Read the model definition and answer for the solid it produces. Units are mm, in the model's axes. Face numbers are marked on the shaded views. A direction names the side the tool comes from. Round coordinates to 2 decimals unless told otherwise and drop trailing zeros. Write each loop counter-clockwise with the first axis right and the second up, starting at its lowest first coordinate (ties: lowest second). Pieces come first, ordered by that corner, then holes.
Autodesk Inventor part; units mm, degrees
ref_plane "YZ Plane" through (0, 0, 0) normal (1, 0, 0) x (0, 1, 0)
ref_plane "XZ Plane" through (0, 0, 0) normal (0, 1, 0) x (-1, 0, 0)
ref_plane "XY Plane" through (0, 0, 0) normal (0, 0, 1) x (1, 0, 0)
sketch "Sketch1" plane through (0, 0, 0) normal (0, 0, 1) x (1, 0, 0)
  line L0 (-91, 0) -> (91, 0) construction
  line L1 (0, -94.2771) -> (0, 159.6624) construction
  circle A0 centre (-30, 27.5) radius 6
  circle A1 centre (30, 27.5) radius 6
  line L2 (-30, 27.5) -> (30, 27.5) construction
  line L3 (30, 27.5) -> (30, -27.5) construction
  line L4 (30, -27.5) -> (-30, -27.5) construction
  line L5 (-30, -27.5) -> (-30, 27.5) construction
  circle A2 centre (-30, -27.5) radius 6
  circle A3 centre (30, -27.5) radius 6
  line L6 (-30, 17.5) -> (-5, 17.5)
  line L7 (-5, 17.5) -> (-5, -17.5)
  line L8 (-5, -17.5) -> (-30, -17.5)
  circle A4 centre (-30, 0) radius 5
  circle A5 centre (-13, 7.5) radius 5.5
  circle A6 centre (-13, -7.5) radius 5.5
  line L9 (-45, 36) -> (45, 36)
  line L10 (45, 36) -> (45, -36)
  line L11 (45, -36) -> (-45, -36)
  line L12 (-45, -36) -> (-45, 36)
  circle A7 centre (-28.9, 45.5) radius 9.25
  circle A8 centre (28.9, 45.5) radius 9.25
  circle A9 centre (-28.9, -45.5) radius 9.25 construction
  circle A10 centre (28.9, -45.5) radius 9.25 construction
  line L13 (-30, 17.5) -> (-35, 17.5)
  line L14 (-35, 17.5) -> (-35, -17.5)
  line L15 (-35, -17.5) -> (-30, -17.5)
  line L16 (-45, 58) -> (45, 58)
  line L17 (45, 58) -> (45, 36)
  line L18 (45, 36) -> (-45, 36)
  line L19 (-45, 36) -> (-45, 58)
  line L20 (-45, -36) -> (45, -36)
  line L21 (45, -36) -> (45, -58) construction
  line L22 (45, -58) -> (-45, -58) construction
  line L23 (-45, -58) -> (-45, -36) construction
  line L24 (-45, -36) -> (-65, -36)
  line L25 (-65, -36) -> (-65, 58)
  line L26 (-65, 58) -> (-45, 58)
  line L27 (-45, 58) -> (-45, -36)
  line L28 (65, -36) -> (45, -36)
  line L29 (45, -36) -> (45, 58)
  line L30 (45, 58) -> (65, 58)
  line L31 (65, 58) -> (65, -36)
  line L32 (-51, -36) -> (-59, -36)
  line L33 (-59, -36) -> (-59, 58)
  line L34 (-59, 58) -> (-51, 58)
  line L35 (-51, 58) -> (-51, -36)
  line L36 (51, -36) -> (59, -36)
  line L37 (59, -36) -> (59, 58)
  line L38 (59, 58) -> (51, 58)
  line L39 (51, 58) -> (51, -36)
  point P0 (0, 0)
  point P1 (-55, 58)
  point P2 (55, 58)
  dimension "d2" = 12
  dimension "d3" = 60
  dimension "d4" = 55
  dimension "d5" = 10
  dimension "d6" = 25
  dimension "d7" = 10
  dimension "d8" = 17
  dimension "d9" = 11
  dimension "d10" = 15
  dimension "d12" = 18
  dimension "d13" = 18.5
  dimension "d14" = 90
  dimension "d15" = 72
  dimension "d18" = 30
  dimension "d25" = 10
  dimension "d26" = 10
  dimension "d28" = 22
  dimension "d35" = 57.8
  dimension "d36" = 20
  dimension "d37" = 8
extrude "Extrusion1" add sketch "Sketch1" against normal blind 10 contours A0 | A1 | A2 | A3 | A4 | L6 L7 L8 L15 L14 L13 | A5 | A6 | L19 L16 L17 L9 | L9 L10 L11 L12 | L12 L24 L35 L26 L19 | L17 L30 L39 L28 L10 | L24 L33 L26 L35 | L39 L30 L37 L28 | L24 L25 L26 L33 | L37 L30 L31 L28
extrude "Extrusion3" cut sketch "Sketch1" against normal through all contours A0 | A1 | A2 | A3
sketch "Sketch2" plane through (0, 0, 0) normal (0, 0, 1) x (1, 0, 0)
  line L0 (-78.9863, 0) -> (78.9863, 0)
  line L1 (0, -92.6147) -> (0, 159.3853)
  line L2 (-56.4188, 123.3853) -> (56.4188, 123.3853)
  line L3 (56.4188, 123.3853) -> (56.4188, 99.2325)
  line L4 (56.4188, -56.6147) -> (-56.4188, -56.6147)
  line L5 (-56.4188, -56.6147) -> (-56.4188, 99.2325)
  line L6 (-56.4188, 99.2325) -> (56.4188, 99.2325)
  line L7 (56.4188, 99.2325) -> (56.4188, -56.6147)
  line L8 (-56.4188, 99.2325) -> (-56.4188, 123.3853)
  point P0 (0, 0)
  dimension "d27" = 180
extrude "Extrusion4" cut sketch "Sketch1" against normal through all contours A4 | A5 | A6
extrude "Extrusion5" cut sketch "Sketch1" against normal through all contours L6 L7 L8 L15 L14 L13
mirror "Mirror2" about plane through (0, 0, 0) normal (1, 0, 0) of "Extrusion4", "Extrusion5"
fillet "Fillet4" radius 5 8 edges at (-35, 17.5, -5) (-5, 17.5, -5) (-35, -17.5, -5) (-5, -17.5, -5) (5, -17.5, -5) (5, 17.5, -5) (35, 17.5, -5) (35, -17.5, -5)
extrude "Extrusion6" cut sketch "Sketch1" against normal blind 6 contours L24 L33 L26 L35 | L39 L30 L37 L28
fillet "Fillet5" radius 5 4 edges at (-65, -36, -5) (65, -36, -5) (65, 58, -5) (-65, 58, -5)
properties part number "z plate bracket"
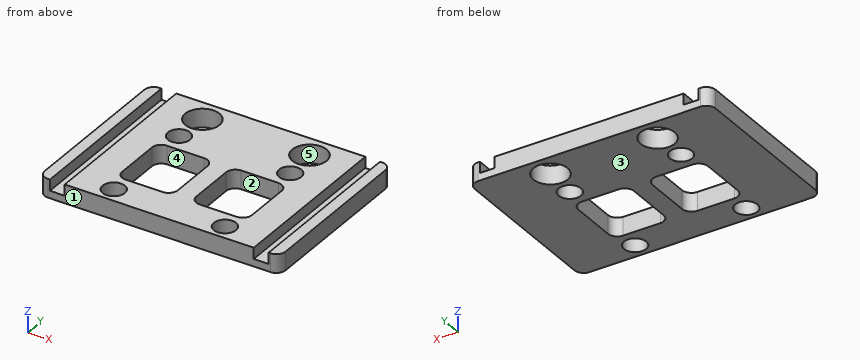
Q1. Which of the six approach directions +Z, -Z, +X, -X, +Y, -Y give full straight-line access (tool end or side, diameter ignored) to the marked faces 1 and 2?
Verdict:
face 1: +Z, -Z, +X, -X, -Y
face 2: +Z, -Z
Q2. Section A-A (z = -8.5) is taken. State how many separate pieces and enclosed holes the cut face has, then the cut area to 3 significant figures.
Verdict:
separate pieces: 1
enclosed holes: 8
area: 9,150 mm2
Q3. Section B-B (y = 27.5) is taken. Determine the outline of the cut face in (x, z).
Verdict:
outline: (-65, -10) - (-36, -10) - (-36, 0) - (-51, 0) - (-51, -6) - (-59, -6) - (-59, 0) - (-65, 0) - close; (-24, -10) - (24, -10) - (24, 0) - (-24, 0) - close; (36, -10) - (65, -10) - (65, 0) - (59, 0) - (59, -6) - (51, -6) - (51, 0) - (36, 0) - close
Q4. Straight lines are drawn through the part: probe 1 along X at (y, z) = (2, -4.25); probe 2 along Y at (x, z) = (-10, -6); probe 3 along Y at (x, z) = (34, -6). For each, find the intervals that lie inside material, in ascending order.
Verdict:
probe 1: x = -65 to -59, -51 to -35, -5 to 5, 35 to 51, 59 to 65
probe 2: y = -36 to -17.5, 17.5 to 58
probe 3: y = -36 to -31.97, -23.03 to -15.5, 15.5 to 23.03, 31.97 to 37.78, 53.22 to 58
Q5. Determine the mould class of the marked faces 3, 4 and 5 for opening direction X: pulls with the +X half, pulls with the -X half, needs draft (parallel to the pull), parting line crosses it, or undercut.
Verdict:
face 3: needs draft
face 4: undercut
face 5: undercut
Q6. Section D-D (y = 38) is taken. Determine the outline of the cut face in (x, z), then the cut area to 3 significant figures.
Verdict:
outline: (-65, -10) - (-34.31, -10) - (-34.31, 0) - (-51, 0) - (-51, -6) - (-59, -6) - (-59, 0) - (-65, 0) - close; (-23.49, -10) - (23.49, -10) - (23.49, 0) - (-23.49, 0) - close; (34.31, -10) - (65, -10) - (65, 0) - (59, 0) - (59, -6) - (51, -6) - (51, 0) - (34.31, 0) - close
area: 987 mm2
